```python
from build123d import *

# Parameters (mm, degrees)
SKETCH1_R           = 225
BOSS_EXTRUDE1_DEPTH = 8
SKETCH2_R           = 5.25
CUT_EXTRUDE1_DEPTH  = 319.298601945
CIRPATTERN1_COUNT   = 16
SKETCH3_R           = 14
BOSS_EXTRUDE2_DEPTH = 15
SKETCH4_R           = 7.5
CUT_EXTRUDE2_DEPTH  = 320.028211919
SKETCH5_R           = 14
BOSS_EXTRUDE3_DEPTH = 15
SKETCH6_R           = 7.5
CUT_EXTRUDE3_DEPTH  = 320.028211919
BOSS_EXTRUDE4_DEPTH = 12.5
FILLET1_R           = 3


with BuildPart() as part:
    # Sketch1 → Boss-Extrude1 (new body)
    with BuildSketch(Plane(origin=(0, 0, 0), x_dir=(1, 0, 0), z_dir=(0, 1, 0))):
        with Locations(Location((0, 0, 0), (0, 0, 270))):
            Circle(SKETCH1_R)
    extrude(amount=BOSS_EXTRUDE1_DEPTH)

    # Sketch2 → Cut-Extrude1 (cut, through all)
    with BuildSketch(Plane(origin=(0, 8, 0), x_dir=(1, 0, 0), z_dir=(0, 1, 0))):
        with Locations(Location((0, 210, 0), (0, 0, 270))):
            Circle(SKETCH2_R)
    cut_extrude1 = extrude(amount=-CUT_EXTRUDE1_DEPTH, mode=Mode.SUBTRACT)

    # CirPattern1: Cut-Extrude1 ×16 about axis
    cirpattern1_axis = Axis((0, 0, 0.114395615), (0, 1, 0))
    for i in range(1, CIRPATTERN1_COUNT):
        add(cut_extrude1.rotate(cirpattern1_axis, i * 360 / CIRPATTERN1_COUNT), mode=Mode.SUBTRACT)

    # Sketch3 → Boss-Extrude2 (add)
    with BuildSketch(Plane(origin=(0, 8, 0), x_dir=(1, 0, 0), z_dir=(0, 1, 0))):
        with Locations(Location((-130, 0, 0), (0, 0, 270))):
            Circle(SKETCH3_R)
    extrude(amount=BOSS_EXTRUDE2_DEPTH)

    # Sketch4 → Cut-Extrude2 (cut, through all)
    with BuildSketch(Plane(origin=(0, 23, 0), x_dir=(1, 0, 0), z_dir=(0, 1, 0))):
        with Locations(Location((-130, 0, 0), (0, 0, 270))):
            Circle(SKETCH4_R)
    extrude(amount=-CUT_EXTRUDE2_DEPTH, mode=Mode.SUBTRACT)

    # Sketch5 → Boss-Extrude3 (add)
    with BuildSketch(Plane(origin=(0, 8, 0), x_dir=(1, 0, 0), z_dir=(0, 1, 0))):
        with Locations(Location((130, 0, 0), (0, 0, 270))):
            Circle(SKETCH5_R)
    extrude(amount=BOSS_EXTRUDE3_DEPTH)

    # Sketch6 → Cut-Extrude3 (cut, through all)
    with BuildSketch(Plane(origin=(0, 23, 0), x_dir=(1, 0, 0), z_dir=(0, 1, 0))):
        with Locations(Location((130, 0, 0), (0, 0, 270))):
            Circle(SKETCH6_R)
    extrude(amount=-CUT_EXTRUDE3_DEPTH, mode=Mode.SUBTRACT)

    # Sketch7 → Boss-Extrude4 (add, symmetric)
    with BuildSketch(Plane.XY):
        Polygon((-106, 8), (-106, 14), (-56, 14), (-56, 108), (56, 108), (56, 14), (106, 14), (106, 8), (50, 8), (50, 102), (-50, 102), (-50, 8), align=None)
    extrude(amount=BOSS_EXTRUDE4_DEPTH, both=True)

    # Fillet1
    fillet1_edges = [part.edges().sort_by_distance(p)[0] for p in [
        (-50, 102, 0),
        (50, 102, 0),
        (106, 14, 0),
        (56, 14, 0),
        (56, 108, 0),
        (-56, 108, 0),
        (-56, 14, 0),
        (-106, 14, 0),
    ]]
    fillet(fillet1_edges, radius=FILLET1_R)


solid = part.part
```
Geometry: final body of the model. Coordinates: model frame, mm. A direction names the side the tool comes from. Give positions to 0.01 mm unless a question says otherwise; leave off trailing zeros. Loops run counter-clockwise (first coordinate to the right, second up) from the corner with the lowest first, then second, coordinate; pieces in that order, holes last. Notation, with made-up numbers: (16.5, 83.5) -> (56.5, 83.5) arc R13 ccw to (56.5, 106.5) -> close; hole circle Ø2 at (-25, 62.25). An arc over 180 degrees is marked (long way). Return JSON: item names as keys, results as strings.
Item 1: Section A-A, the plane y = 79.5. Output: boundary loops of the cut face in (x, z), plus the area to 3 significant figures.
Filled in:
{"outline": "(-56, -12.5) -> (-50, -12.5) -> (-50, 12.5) -> (-56, 12.5) -> close; (50, -12.5) -> (56, -12.5) -> (56, 12.5) -> (50, 12.5) -> close", "area": "300 mm^2"}
Item 2: Section C-C, the plane z = -210. Output: boundary loops of the cut face in (x, y).
Filled in:
{"outline": "(-80.78, 0) -> (-5.25, 0) -> (-5.25, 8) -> (-80.78, 8) -> close; (5.25, 0) -> (80.78, 0) -> (80.78, 8) -> (5.25, 8) -> close"}
Item 3: Section D-D, the plane x = -130. Output: boundary loops of the cut face in (y, z), plus the area to 3 significant figures.
Filled in:
{"outline": "(0, -183.64) -> (8, -183.64) -> (8, -14) -> (23, -14) -> (23, -7.5) -> (0, -7.5) -> close; (0, 7.5) -> (23, 7.5) -> (23, 14) -> (8, 14) -> (8, 183.64) -> (0, 183.64) -> close", "area": "3,010 mm^2"}
Item 4: Mould query, pull axis Z, two halves, no side actions, for faces 5 (the flat face through (124, 23, 6)), 6 (the cylindrical face through (-132.87, 11.66, 6.93)), 7 (the cylindrical face through (-116.12, 15.4, -1.82)). Classes: released by +Z, released by -Z, zero draft, split by the parting line, or undercut.
Filled in:
{"face 5": "zero draft", "face 6": "undercut", "face 7": "split by the parting line"}
Item 5: Section B-B, the plane x = 0. Output: boundary loops of the cut face in (y, z).
Filled in:
{"outline": "(0, -225) -> (8, -225) -> (8, -215.25) -> (0, -215.25) -> close; (0, -204.75) -> (8, -204.75) -> (8, 204.98) -> (0, 204.98) -> close; (0, 215.48) -> (8, 215.48) -> (8, 225) -> (0, 225) -> close; (102, -12.5) -> (108, -12.5) -> (108, 12.5) -> (102, 12.5) -> close"}
Item 6: Line query: line 1 (Y direction, x = -8.5, z = 2); line 2 (X direction, y = 5.75, z = 0); line 3 (Y direction, x = -112, z = 128.5). Output: solid intervals per line, ascending.
Filled in:
{"line 1": "0 to 8, 102 to 108", "line 2": "-225 to -215.36, -204.87 to -137.5, -122.5 to 122.5, 137.5 to 204.87, 215.36 to 225", "line 3": "0 to 8"}
Item 7: Pin query (flat end, axial travel): P1, Ø17, axis at x = -148.57, z = -148.46, coming from the +Y side; P2, Ø8, axis at y = 39, z = -12.5, coming from the -X side; P3, Ø1.5, axis at y = 10, z = -2.5, coming from the -X side; P4, Ø13.5, axis at x = 130, z = 0, coming from the -Y side. Return the tip coordinate at first contact, or that it passes through.
Filled in:
{"P1": "y = 8", "P2": "x = -56", "P3": "x = -143.89", "P4": "through"}
Item 8: Access query for faces 1 (the flat face through (81, 14, 0)), 2 (the flat face through (8, 103, 12.5)), 3 (the flat face through (50, 53, 0)), 4 (the cylindrical face through (143.88, 15.4, -1.82)). Directions: +Z, -Z, +X, -X, +Y, -Y. A direction counts if a zero-diameter tool reaches every point of the face in a straight line with its end or side. Return the directions, or none.
Filled in:
{"face 1": "+Z, -Z, +Y", "face 2": "+Z, +Y", "face 3": "+Z, -Z", "face 4": "+Y"}
